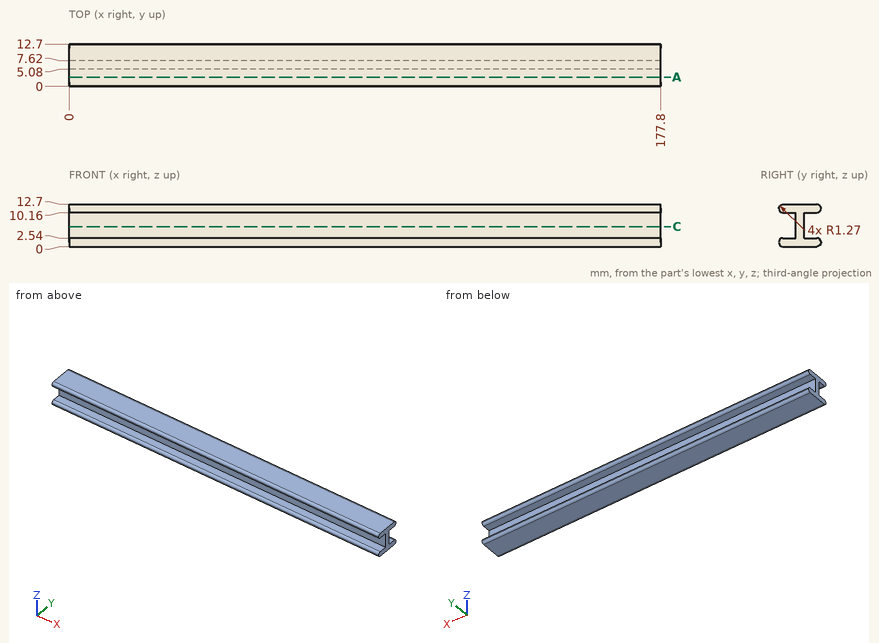
Print and shaded views of the part. All mm, measured from the part's lowest x, y and z. Give positions to 0.01 mm unless a question says otherwise; leave off trailing zeros. Loops run counter-clockwise (first coordinate to the right, second up) from the corner with the lowest first, then second, coordinate; pieces in that order, holes last. Notation, with made-up numbers: (4.5, 45) - (20.5, 45) arc R17 cw to (20.5, 69) - close; hole circle Ø11 at (73.5, -35). An arc over 180 degrees is marked (long way). Use a Markdown table: item, result.
(1) Band-saw the part on C-C (z = 6). Give the cut face in (x, y), and give its area (3 significant figures).
Taken from the geometry:
| item | result |
|---|---|
| outline | (0, 5.08) - (177.8, 5.08) - (177.8, 7.62) - (0, 7.62) - close |
| area | 452 mm2 |
(2) Wall check: line 1 along Z through (x, y) = (97.5, 7.75); line 2 along Y through (x, z) = (67.5, 5.5); line 3 along Z through (x, y) = (169, 0.75). Give the ranges that are in metal, low to high.
Taken from the geometry:
| item | result |
|---|---|
| line 1 | 0 to 2.54, 10.16 to 12.7 |
| line 2 | 5.08 to 7.62 |
| line 3 | 0.11 to 2.43, 10.27 to 12.59 |
(3) Band-saw the part on A-A (y = 2.75). Give the cut face in (x, z), and give its area (3 significant figures).
Taken from the geometry:
| item | result |
|---|---|
| outline | (0, 0) - (177.8, 0) - (177.8, 2.54) - (0, 2.54) - close; (0, 10.16) - (177.8, 10.16) - (177.8, 12.7) - (0, 12.7) - close |
| area | 903 mm2 |
(4) Drop flat-ended pins along their axis: pin 1 Ø5 at (x, z) = (113, 8) entering from -Y; pin 2 Ø2.5 at (x, z) = (108.5, 7.5) entering from +Y; pin 3 Ø1.5 at (x, z) = (149.5, 10.5) entering from +Y. Give the stop position or say it passes through.
Taken from the geometry:
| item | result |
|---|---|
| pin 1 | y = 0.41 |
| pin 2 | y = 7.62 |
| pin 3 | y = 12.69 |
